Could you check a few things on this model? Use its own coordinates, in mm. A direction names the side the tool comes from. Coordinates: 2 decimals unless noted, no trailing zeros. Loops run counter-clockwise (first coordinate to the right, second up) from the corner with the lowest first, then second, coordinate; pieces in that order, holes last.
from build123d import *

# Parameters (mm, degrees)
SKETCH_1_R      = 2.2
SKETCH_1_R_2    = 2.5
EXTRUDE_1_DEPTH = 2


with BuildPart() as part:
    # 草图1 → 凸台-拉伸1 (new body)
    with BuildSketch(Plane(origin=(0, 0, 0), x_dir=(1, 0, 0), z_dir=(0, 1, 0))):
        Polygon((159.754738648, 48.995603023), (150.004738648, 48.995603023), (150.004738648, 46.495603023), (151.504738648, 46.495603023), (151.504738648, 43.895603023), (150.004738648, 43.895603023), (150.004738648, 40.895603023), (147.004738648, 40.895603023), (147.004738648, 43.895603023), (145.504738648, 43.895603023), (145.504738648, 46.495603023), (147.004738648, 46.495603023), (147.004738648, 48.995603023), (138.604738648, 48.995603023), (133.504738648, 48.995603023), (118.504738648, 48.995603023), (118.504738648, 33.995603023), (118.504738648, 21.495603023), (118.504738648, 20.495603023), (121.004738648, 20.495603023), (121.004738648, 21.995603023), (123.604738648, 21.995603023), (123.604738648, 20.495603023), (126.604738648, 20.495603023), (126.604738648, 17.495603023), (123.604738648, 17.495603023), (123.604738648, 15.995603023), (121.004738648, 15.995603023), (121.004738648, 17.495603023), (118.504738648, 17.495603023), (118.504738648, 7.745603023), (116.504738648, 7.745603023), (116.504738648, -0.254396977), (118.504738648, -0.254396977), (118.504738648, -27.754396977), (116.504738648, -27.754396977), (116.504738648, -35.754396977), (118.504738648, -35.754396977), (118.504738648, -45.504396977), (121.004738648, -45.504396977), (121.004738648, -44.004396977), (123.604738648, -44.004396977), (123.604738648, -45.504396977), (126.604738648, -45.504396977), (126.604738648, -48.504396977), (123.604738648, -48.504396977), (123.604738648, -50.004396977), (121.004738648, -50.004396977), (121.004738648, -48.504396977), (118.504738648, -48.504396977), (118.504738648, -56.904396977), (118.504738648, -62.004396977), (118.504738648, -77.004396977), (133.504738648, -77.004396977), (146.004738648, -77.004396977), (147.004738648, -77.004396977), (147.004738648, -74.504396977), (145.504738648, -74.504396977), (145.504738648, -71.904396977), (147.004738648, -71.904396977), (147.004738648, -68.904396977), (150.004738648, -68.904396977), (150.004738648, -71.904396977), (151.504738648, -71.904396977), (151.504738648, -74.504396977), (150.004738648, -74.504396977), (150.004738648, -77.004396977), (159.754738648, -77.004396977), (159.754738648, -79.004396977), (167.754738648, -79.004396977), (167.754738648, -77.004396977), (195.254738648, -77.004396977), (195.254738648, -79.004396977), (203.254738648, -79.004396977), (203.254738648, -77.004396977), (213.004738648, -77.004396977), (213.004738648, -74.504396977), (211.504738648, -74.504396977), (211.504738648, -71.904396977), (213.004738648, -71.904396977), (213.004738648, -68.904396977), (216.004738648, -68.904396977), (216.004738648, -71.904396977), (217.504738648, -71.904396977), (217.504738648, -74.504396977), (216.004738648, -74.504396977), (216.004738648, -77.004396977), (224.404738648, -77.004396977), (229.504738648, -77.004396977), (244.504738648, -77.004396977), (244.504738648, -62.004396977), (244.504738648, -49.504396977), (244.504738648, -48.504396977), (242.004738648, -48.504396977), (242.004738648, -50.004396977), (239.404738648, -50.004396977), (239.404738648, -48.504396977), (236.404738648, -48.504396977), (236.404738648, -45.504396977), (239.404738648, -45.504396977), (239.404738648, -44.004396977), (242.004738648, -44.004396977), (242.004738648, -45.504396977), (244.504738648, -45.504396977), (244.504738648, -35.754396977), (246.504738648, -35.754396977), (246.504738648, -27.754396977), (244.504738648, -27.754396977), (244.504738648, -0.254396977), (246.504738648, -0.254396977), (246.504738648, 7.745603023), (244.504738648, 7.745603023), (244.504738648, 17.495603023), (242.004738648, 17.495603023), (242.004738648, 15.995603023), (239.404738648, 15.995603023), (239.404738648, 17.495603023), (236.404738648, 17.495603023), (236.404738648, 20.495603023), (239.404738648, 20.495603023), (239.404738648, 21.995603023), (242.004738648, 21.995603023), (242.004738648, 20.495603023), (244.504738648, 20.495603023), (244.504738648, 28.895603023), (244.504738648, 33.995603023), (244.504738648, 48.995603023), (229.504738648, 48.995603023), (217.004738648, 48.995603023), (216.004738648, 48.995603023), (216.004738648, 46.495603023), (217.504738648, 46.495603023), (217.504738648, 43.895603023), (216.004738648, 43.895603023), (216.004738648, 40.895603023), (213.004738648, 40.895603023), (213.004738648, 43.895603023), (211.504738648, 43.895603023), (211.504738648, 46.495603023), (213.004738648, 46.495603023), (213.004738648, 48.995603023), (203.254738648, 48.995603023), (203.254738648, 50.995603023), (195.254738648, 50.995603023), (195.254738648, 48.995603023), (167.754738648, 48.995603023), (167.754738648, 50.995603023), (159.754738648, 50.995603023), align=None)
        with Locations(Location((181.504738648, -56.504396977, 0), (0, 0, 270))):
            Circle(SKETCH_1_R, mode=Mode.SUBTRACT)
        with Locations(Location((139.004738648, -14.004396977, 0), (0, 0, 270))):
            Circle(SKETCH_1_R, mode=Mode.SUBTRACT)
        with Locations(Location((211.556776849, 16.047641223, 0), (0, 0, 270))):
            Circle(SKETCH_1_R, mode=Mode.SUBTRACT)
        with Locations(Location((181.504738648, 28.49819903, 0), (0, 0, 270))):
            Circle(SKETCH_1_R, mode=Mode.SUBTRACT)
        with Locations(Location((151.452700448, -44.056435178, 0), (0, 0, 270))):
            Circle(SKETCH_1_R_2, mode=Mode.SUBTRACT)
        with BuildLine():
            Line((223.189738648, -11.79024286), (224.819738648, -11.79024286))
            ThreePointArc((224.819738648, -11.79024286), (227.033892766, -14.004396977), (224.819738648, -16.218551095))
            Line((224.819738648, -16.218551095), (223.189738648, -16.218551095))
            ThreePointArc((223.189738648, -16.218551095), (220.975584531, -14.004396977), (223.189738648, -11.79024286))
        make_face(mode=Mode.SUBTRACT)
        with BuildLine():
            ThreePointArc((156.373636186, -43.170776407), (154.281127573, -41.228008053), (152.338359218, -39.135499439))
            ThreePointArc((152.338359218, -39.135499439), (136.585624733, -32.610503171), (143.110621001, -16.857768685))
            ThreePointArc((143.110621001, -16.857768685), (143.004738648, -14.004396977), (143.110621001, -11.15102527))
            ThreePointArc((143.110621001, -11.15102527), (143.110621001, 24.38972067), (178.65136694, 24.38972067))
            ThreePointArc((178.65136694, 24.38972067), (181.504738648, 24.495603023), (184.358110356, 24.38972067))
            ThreePointArc((184.358110356, 24.38972067), (200.110844842, 30.914716938), (206.63584111, 15.161982452))
            ThreePointArc((206.63584111, 15.161982452), (208.728349724, 13.219214098), (210.671118078, 11.126705484))
            ThreePointArc((210.671118078, 11.126705484), (226.423852564, 4.601709216), (219.898856295, -11.15102527))
            ThreePointArc((219.898856295, -11.15102527), (220.004738648, -14.004396977), (219.898856295, -16.857768685))
            ThreePointArc((219.898856295, -16.857768685), (219.898856295, -52.398514625), (184.358110356, -52.398514625))
            ThreePointArc((184.358110356, -52.398514625), (181.504738648, -52.504396977), (178.65136694, -52.398514625))
            ThreePointArc((178.65136694, -52.398514625), (162.898632455, -58.923510893), (156.373636186, -43.170776407))
        make_face(mode=Mode.SUBTRACT)
    extrude(amount=EXTRUDE_1_DEPTH)


solid = part.part
1) Imagine slicing it at A-A on x = 201.5. List the corners of the cut face in (y, z) for me.
2) If I drill on L1, parallel to X at y = 1.05, z = -41.5; L2, parallel to X at y = 1.25, z = 14; L3, parallel to X at y = 1.95, z = 45, over which ranges is the centre line in solid material (lowest first)?
3) Will these pins go through, and if not, where does the flat tip stop? pin 1 (0.6 mm diameter, centred on x = 208.5, y = 1.5, fed in from +Z); pin 2 (0.6 mm diameter, centred on x = 186.5, y = 1.5, fed in from -Z); pin 3 (0.6 mm diameter, centred on y = 1, z = 47, fed in from +X).
4) Imagine slicing it at B-B on y = 1.35. State how many separate pieces and enclosed holes the cut face has, plus the area to 3 significant figures.
5) For faces 1 (the flat face through (137, 2, -16)), 2 (the cylindrical face through (154.309, 0.986, 41.256)), which set-ups out of +Z, -Z, +X, -X, +Y, -Y let a thin tool reach every point of the face, with its end or its side?
6) We'd pull the mould along X, two halves only. Please class faces 3 (the flat face through (137, 0, -16)), 4 (the cylindrical face through (208.7, 0.99, -13.25)): released by +X, released by -X, zero draft, split by the parting line, or undercut.
7) Imagine slicing it at C-C on x = 231.5. List the corners of the cut face in (y, z) for me, plus the area to 3 significant figures.
Solved:
1. outline: (0, -51) - (2, -51) - (2, -30.23) - (0, -30.23) - close; (0, 59.75) - (2, 59.75) - (2, 79) - (0, 79) - close
2. L1: x = 118.5 to 147, 150 to 213, 216 to 244.5
2. L2: x = 118.5 to 136.8, 141.2 to 143, 220 to 220.98, 227.03 to 244.5
2. L3: x = 118.5 to 121, 123.6 to 149.14, 153.77 to 155.78, 225.02 to 239.4, 242 to 244.5
3. pin 1: stops at z = 77
3. pin 2: stops at z = -49
3. pin 3: stops at x = 236.4
4. separate pieces: 1
4. enclosed holes: 7
4. area: 8,860 mm2
5. face 1: +Z, -Z, +X, -X, +Y
5. face 2: +Y, -Y
6. face 3: zero draft
6. face 4: undercut
7. outline: (0, -49) - (2, -49) - (2, 77) - (0, 77) - close
7. area: 252 mm2
